Geometry: final body of the model. Coordinates: model frame, mm. Coordinates: 2 decimals unless noted, no trailing zeros. Order: outer loops, then holes, each group sorted by start corner. A loop starts at its lowest first (then second) coordinate and runs counter-clockwise, first axis right, second up. Notation, with made-up numbers: M 32.25,76 L 66.25,76 A23 ccw 66.25,88 Z; hole C 2.25,-16.75 d6. An arc over 180 degrees is marked long. One line per question, with ' | ' between items.
from build123d import *

# Parameters (mm, degrees)
F0_W     = 3
F0_H     = 12
F1_DEPTH = 3


with BuildPart() as f1:
    # F0 (on Front) → F1 (new body)
    with BuildSketch(Plane.XZ):
        with BuildLine():
            Line((10, 24), (10, 15))
            Line((10, 15), (-10, 15))
            Line((-10, 15), (-10, 24))
            Line((-10, 24), (-22, 24))
            Line((-22, 24), (-22, 15))
            Line((-22, 15), (-22, 1))
            Line((-22, 1), (-14, 1))
            ThreePointArc((-14, 1), (-9, -4), (-14, -9))
            Line((-14, -9), (-22, -9))
            Line((-22, -9), (-22, -15))
            Line((-22, -15), (-22, -18))
            Line((-22, -18), (-10, -18))
            Line((-10, -18), (-10, -15))
            Line((-10, -15), (10, -15))
            Line((10, -15), (10, -18))
            Line((10, -18), (22, -18))
            Line((22, -18), (22, -15))
            Line((22, -15), (22, -9))
            Line((22, -9), (14, -9))
            ThreePointArc((14, -9), (9, -4), (14, 1))
            Line((14, 1), (22, 1))
            Line((22, 1), (22, 15))
            Line((22, 15), (22, 24))
            Line((22, 24), (10, 24))
        make_face()
        Rectangle(F0_W, F0_H, mode=Mode.SUBTRACT)
    extrude(amount=F1_DEPTH)


solid = f1.part
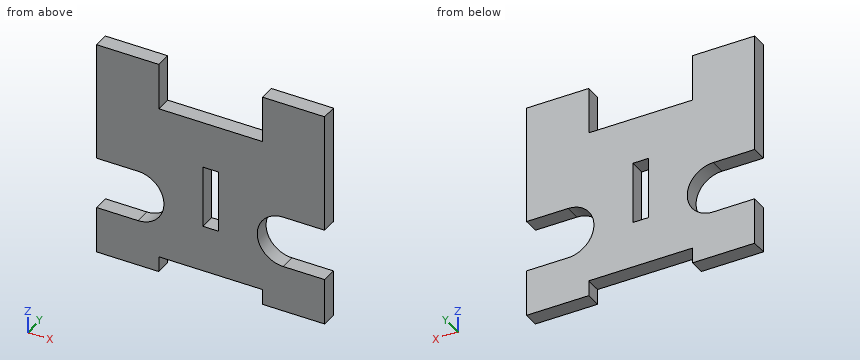
1. Material intervals for line 1 (Z direction, x = -18, y = -2.75); line 2 (X direction, y = -0.6, z = 4); line 3 (X direction, y = -0.9, z = 17), sorted ascending. Write a range as [from, to].
Response values:
line 1: z = [-18, -9], [1, 24] | line 2: x = [-22, -1.5], [1.5, 22] | line 3: x = [-22, -10], [10, 22]
2. Section C-C, the plane z = 19. Output: boundary loops of the cut face in (x, y), and give its area (3 significant figures).
Response values:
outline: M -22,-3 L -10,-3 L -10,0 L -22,0 Z; M 10,-3 L 22,-3 L 22,0 L 10,0 Z | area: 72.0 mm^2
3. Section D-D, the plane x = -6. Output: boundary loops of the cut face in (y, z), and give its area (3 significant figures).
Response values:
outline: M -3,-15 L 0,-15 L 0,15 L -3,15 Z | area: 90.0 mm^2
4. Section B-B, the plane y = -1.8. Output: boundary loops of the cut face in (x, z), and give its area (3 significant figures).
Response values:
outline: M -22,-18 L -10,-18 L -10,-15 L 10,-15 L 10,-18 L 22,-18 L 22,-9 L 14,-9 A5 cw 14,1 L 22,1 L 22,24 L 10,24 L 10,15 L -10,15 L -10,24 L -22,24 L -22,1 L -14,1 A5 cw -14,-9 L -22,-9 Z; hole M -1.5,-6 L 1.5,-6 L 1.5,6 L -1.5,6 Z | area: 1,330 mm^2
5. Section A-A, the plane z = -1. Output: boundary loops of the cut face in (x, y), and give its area (3 significant figures).
Response values:
outline: M -10,-3 L -1.5,-3 L -1.5,0 L -10,0 Z; M 1.5,-3 L 10,-3 L 10,0 L 1.5,0 Z | area: 51.0 mm^2
6. Pin query (flat end, axial travel): P1, Ø1.5, axis at x = -1.5, y = -1.5, coming from the -Z side; P2, Ø1.5, axis at x = 0, y = -1, coming from the +Z side. Return the tip coordinate at first contact, or that it passes through.
Response values:
P1: stops at z = -15 | P2: stops at z = 15
